```python
from build123d import *

# Parameters (mm, degrees)
BOSS_EXTRUDE1_DEPTH = 500
FILLET1_R           = 10
BOSS_EXTRUDE2_DEPTH = 26


with BuildPart() as part:
    # Sketch1 → Boss-Extrude1 (new body)
    with BuildSketch(Plane(origin=(0, 0, 0), x_dir=(1, 0, 0), z_dir=(0, 1, 0))):
        with BuildLine():
            Line((-566.6, 0), (-1066.6, 0))
            ThreePointArc((-1066.6, 0), (0, 1066.6), (1066.6, 0))
            Line((1066.6, 0), (566.6, 0))
            ThreePointArc((566.6, 0), (0, 566.6), (-566.6, 0))
        make_face()
    extrude(amount=BOSS_EXTRUDE1_DEPTH)

    # Fillet1
    fillet1_edges = [part.edges().sort_by_distance(p)[0] for p in [
        (0, 500, -1066.6),
        (0, 500, -566.6),
        (0, 0, -1066.6),
        (0, 0, -566.6),
    ]]
    fillet(fillet1_edges, radius=FILLET1_R)

    # Sketch2 → Cut-Revolve1 (revolve, cut)
    with BuildSketch(Plane.XY):
        with BuildLine():
            Line((-1066.6, 216), (-566.6, 216))
            Line((-566.6, 216), (-566.6, 0))
            Line((-566.6, 0), (-1145.861102691, 0))
            Line((-1145.861102691, 0), (-1145.861102691, 500))
            Line((-1145.861102691, 500), (-782.6, 500))
            ThreePointArc((-782.6, 500), (-983.418325857, 416.818325857), (-1066.6, 216))
        make_face()
    revolve(axis=Axis((0, 0, 0), (0, 1, 0)), mode=Mode.SUBTRACT)

    # Sketch3 → Boss-Extrude2 (add)
    with BuildSketch(Plane.XY):
        with BuildLine():
            Line((-782.6, 500), (-576.6, 500))
            ThreePointArc((-576.6, 500), (-569.528932188, 497.071067812), (-566.6, 490))
            Line((-566.6, 490), (-566.6, 216))
            Line((-566.6, 216), (-1066.6, 216))
            ThreePointArc((-1066.6, 216), (-983.418325857, 416.818325857), (-782.6, 500))
        make_face()
        with BuildLine():
            Line((576.6, 500), (782.6, 500))
            ThreePointArc((782.6, 500), (983.418325857, 416.818325857), (1066.6, 216))
            Line((1066.6, 216), (566.6, 216))
            Line((566.6, 216), (566.6, 490))
            ThreePointArc((566.6, 490), (569.528932188, 497.071067812), (576.6, 500))
        make_face()
    extrude(amount=BOSS_EXTRUDE2_DEPTH)


solid = part.part
```
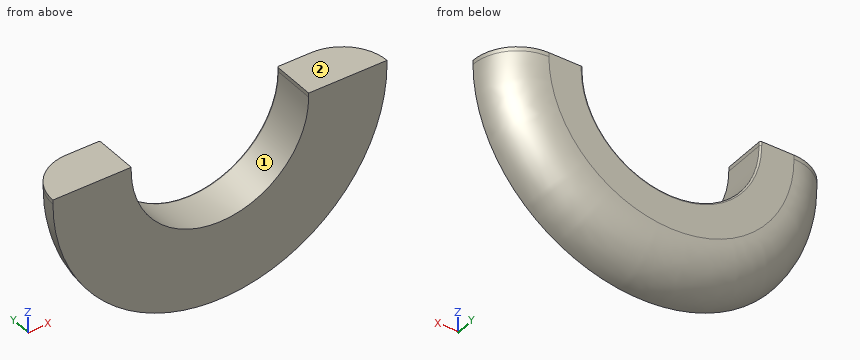
Here's how the part is built. I have some questions about the finished solid (model axes, mm). Face numbers are marked on the shaded views. Coordinates: 2 decimals unless noted, no trailing zeros. Order: outer loops, then holes, each group sorted by start corner. A loop starts at its lowest first (then second) coordinate and runs counter-clockwise, first axis right, second up.
Item 1: If we section it at B-B, the plane y = 345: List the corners of the cut face in (x, z) for me.
Response values:
outline: (-1035.61, 0) arc R1035.61 ccw to (1035.61, 0) - (1035.61, 26) - (566.6, 26) - (566.6, 0) arc R566.6 cw to (-566.6, 0) - (-566.6, 26) - (-1035.61, 26) - close
Item 2: If we section it at A-A, the plane x = 0: List the corners of the cut face in (y, z) for me, then the cut area to 3 significant figures.
Response values:
outline: (216, -1066.6) arc R284 ccw to (500, -782.6) - (500, -576.6) arc R10 ccw to (490, -566.6) - (216, -566.6) - close
area: 125,000 mm2
Item 3: I need wall thicknesses on probe 1 along Y at (x, z) = (314, -733.5); probe 2 along X at (y, z) = (360, -310); probe 3 along Y at (x, z) = (-704.5, -782). Which ranges of each line are inside material? Lowest first, please.
Response values:
probe 1: y = 216 to 499.59
probe 2: x = -979.5 to -474.27, 474.27 to 979.5
probe 3: y = 216 to 304.25
Item 4: Thinking about a two-plate mould opening in X: for the marked faces 1 and 2, which applies, pulls with the +X half, pulls with the -X half, needs draft (parallel to the pull), parting line crosses it, or undercut?
Response values:
face 1: undercut
face 2: needs draft
Item 5: I'm going to push flat-ended pins straight in: pin 1 Ø4 at (x, y) = (-494, 359.5) entering from +Z; pin 2 Ø5 at (x, y) = (417.5, 314.5) entering from +Z; pin 3 Ø3 at (y, z) = (251.5, -313.5) entering from +X. Where does each tip first touch, or does it pass through?
Response values:
pin 1: stops at z = -273.9
pin 2: stops at z = -380.31
pin 3: stops at x = 1017.66
